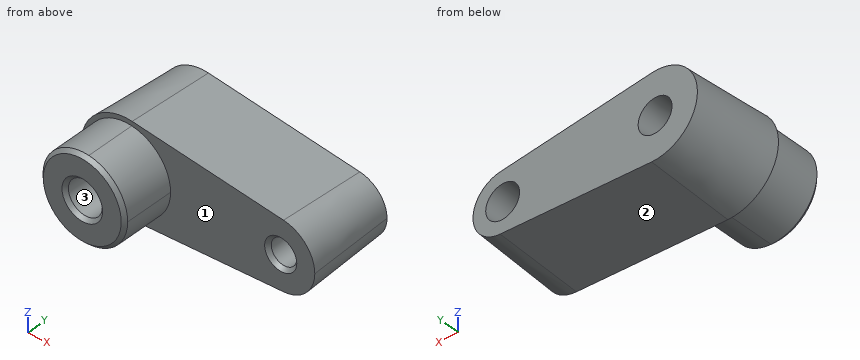
from build123d import *

# Parameters (mm, degrees)
F0_R     = 10
F1_DEPTH = 50
F1_TAPER = -3
F2_DEPTH = 80


# Not quite as in the source:
# - a fillet or chamfer that OpenCascade refuses, or shapes differently, is made with other operations: its cross-section is extruded or revolved along the edge and cut away or added


with BuildPart() as f1:
    # F0 (on Front) → F1 (new body)
    with BuildSketch(Plane.XZ):
        with BuildLine():
            ThreePointArc((2.0833333333, -24.9130432148), (18.3995018048, -16.9250800097), (25, 0))
            ThreePointArc((25, 0), (18.3995018048, 16.9250800097), (2.0833333333, 24.9130432148))
            ThreePointArc((2.0833333333, 24.9130432148), (-25, 0), (2.0833333333, -24.9130432148))
        make_face()
        Circle(F0_R, mode=Mode.SUBTRACT)
        with BuildLine():
            ThreePointArc((2.0833333333, 24.9130432148), (18.3995018048, 16.9250800097), (25, 0))
            ThreePointArc((25, 0), (18.3995018048, -16.9250800097), (2.0833333333, -24.9130432148))
            Line((2.0833333333, -24.9130432148), (91.4583333333, -17.4391302504))
            ThreePointArc((91.4583333333, -17.4391302504), (72.5, 0), (91.4583333333, 17.4391302504))
            Line((91.4583333333, 17.4391302504), (2.0833333333, 24.9130432148))
        make_face()
        with BuildLine():
            ThreePointArc((107.5, 0), (102.8796512634, 11.8475560068), (91.4583333333, 17.4391302504))
            ThreePointArc((91.4583333333, 17.4391302504), (72.5, 0), (91.4583333333, -17.4391302504))
            ThreePointArc((91.4583333333, -17.4391302504), (102.8796512634, -11.8475560068), (107.5, 0))
        make_face()
        with Locations((90, 0)):
            Circle(F0_R, mode=Mode.SUBTRACT)
    extrude(amount=F1_DEPTH, taper=F1_TAPER)

    # F0 (on Front) → F2 (join)
    with BuildSketch(Plane.XZ):
        with BuildLine():
            ThreePointArc((2.0833333333, -24.9130432148), (18.3995018048, -16.9250800097), (25, 0))
            ThreePointArc((25, 0), (18.3995018048, 16.9250800097), (2.0833333333, 24.9130432148))
            ThreePointArc((2.0833333333, 24.9130432148), (-25, 0), (2.0833333333, -24.9130432148))
        make_face()
        Circle(F0_R, mode=Mode.SUBTRACT)
    extrude(amount=F2_DEPTH)

    # F3: chamfer of 2 on 3 edges, made by hand

    # F3_s1 → F3_t2 (revolve, cut)
    with BuildSketch(Plane(origin=(0, 0, 0), x_dir=(0, 1, 0), z_dir=(0.9965217286, 0, 0.0833333333))):
        Polygon((-78, -25), (-80, -23), (-80, -25), align=None)
    revolve(axis=Axis((0, -80, 0), (0, 1, 0)), mode=Mode.SUBTRACT)

    # F3_s3 → F3_t4 (revolve, cut)
    with BuildSketch(Plane.XY):
        Polygon((12, -80), (10, -78), (10, -80), align=None)
    revolve(axis=Axis((0, -80, 0), (0, -1, 0)), mode=Mode.SUBTRACT)

    # F3_s5 → F3_t6 (revolve, cut)
    with BuildSketch(Plane.XY):
        Polygon((99.4871712864, -50), (97.4899122169, -47.8953280875), (97.3796110358, -50), align=None)
    revolve(axis=Axis((90, -50, 0), (0, 1, 0)), mode=Mode.SUBTRACT)


solid = f1.part
Verification items for the finished model (mm, model axes). Face numbers are marked on the shaded views. Coordinates: 2 decimals unless noted, no trailing zeros. Order: outer loops, then holes, each group sorted by start corner. A loop starts at its lowest first (then second) coordinate and runs counter-clockwise, first axis right, second up.
1. Go/stop test with flat-tipped pins: pin 1 Ø8 at (x, y) = (10.5, -43) entering from +Z; pin 2 Ø1 at (y, z) = (-34.5, -3.5) entering from +X; pin 3 Ø1.5 at (x, y) = (7.5, -72) entering from +Z. Record where each tip stops, or that it passes through.
Results found:
pin 1: stops at z = 26.87
pin 2: stops at x = 109.08
pin 3: stops at z = 24.07
2. Sectioned sample at A-A, the plane x = 90. Record the cut outline in (y, z), and give its area (3 significant figures).
Results found:
outline: (-50, -20.19) - (0, -17.56) - (0, -10) - (-47.9, -7.49) - (-50, -9.49) - close; (-50, 9.49) - (-47.9, 7.49) - (0, 10) - (0, 17.56) - (-50, 20.19) - close
area: 1,010 mm2
3. Release check for a two-part mould opening along X. For the marked faces 1, 2 and 3 record: +X half, -X half, draft (parallel to the pull), parting line (faces both ways), or undercut.
Results found:
face 1: draft
face 2: +X half
face 3: undercut
4. Sectioned sample at D-D, the plane z = -6.5. Give the number of separate pieces and of enclosed holes in the cut face, and give its area (3 significant figures).
Results found:
separate pieces: 3
enclosed holes: 0
area: 6,490 mm2
5. Sectioned sample at C-C, the plane y = -12.5. Record the cut outline in (x, z).
Results found:
outline: (2.14, -25.57) - (91.51, -18.09) arc R18.16 ccw to (91.51, 18.09) - (2.14, 25.57) arc R25.66 ccw (long way) to start; hole circle Ø18.69 at (0, 0); hole circle Ø18.69 at (90, 0)
6. Scan lines: line 1 (Z direction, x = 0, y = -57); line 2 (Y direction, x = 72.5, z = -5); line 3 (Z direction, x = 89, y = -16). Record each from-to range of solid material in increasing order.
Results found:
line 1: z = -25 to -10, 10 to 25
line 2: y = -50 to 0
line 3: z = -18.49 to -9.11, 9.11 to 18.49
7. Sectioned sample at B-B, the plane y = -55.5. Record the cut outline in (x, z), and give its area (3 significant figures).
Results found:
outline: circle Ø50 at (0, 0); hole circle Ø20 at (0, 0)
area: 1,650 mm2
